Part model, mm, in its own coordinate system. A direction names the side the tool comes from. Coordinates: 2 decimals unless noted, no trailing zeros. Loops run counter-clockwise (first coordinate to the right, second up) from the corner with the lowest first, then second, coordinate; pieces in that order, holes last. Notation, with made-up numbers: (83, 11.5) - (127, 11.5) arc R14 ccw to (127, 17.5) - close; hole circle Ø6 at (53.5, -19.5). An arc over 180 degrees is marked (long way). Answer as CSV lines item,"result".
from build123d import *

# Parameters (mm, degrees)
SKETCH1_R           = 1.625
BOSS_EXTRUDE1_DEPTH = 5.842


with BuildPart() as part:
    # Sketch1 → Boss-Extrude1 (new body)
    with BuildSketch(Plane(origin=(0, 0, 0), x_dir=(1, 0, 0), z_dir=(0, 1, 0))):
        with BuildLine():
            Line((-23.368, 3.4), (-9.921693404, 3.4))
            ThreePointArc((-9.921693404, 3.4), (-7.818582155, 3.863820652), (-6.105657479, 5.169230769))
            ThreePointArc((-6.105657479, 5.169230769), (8, 0), (-6.105657479, -5.169230769))
            ThreePointArc((-6.105657479, -5.169230769), (-7.818582155, -3.863820652), (-9.921693404, -3.4))
            Line((-9.921693404, -3.4), (-23.368, -3.4))
            ThreePointArc((-23.368, -3.4), (-26.768, 0), (-23.368, 3.4))
        make_face()
        with Locations((-19.304, 0)):
            Circle(SKETCH1_R, mode=Mode.SUBTRACT)
        with Locations((-23.368, 0)):
            Circle(SKETCH1_R, mode=Mode.SUBTRACT)
    extrude(amount=BOSS_EXTRUDE1_DEPTH)


solid = part.part
Q1. Wall check: L1, parallel to X at y = 2.95, z = 0; L2, parallel to Z at x = -10, y = 5.55; L3, parallel to Z at x = -24, y = 0.45. Give the ranges that are in metal, low to high.
Results:
L1,"x = -26.77 to -24.99, -21.74 to -20.93, -17.68 to 8"
L2,"z = -3.4 to 3.4"
L3,"z = -3.34 to -1.5, 1.5 to 3.34"
Q2. Which spindle directions (+Z, -Z, +X, -X, +Y, -Y) get a long thin tool onto all of the face, cutting with end or side? Do faces 1 (the face through (-17, 3, 3.4)), 2 (the face through (-5, 5.842, 0)). Say none if no direction does.
Results:
face 1,"+Z, -X, +Y, -Y"
face 2,"+Z, -Z, +X, -X, +Y"
Q3. Two-plate mould, pull along X, no slides. Class faces 3 (the face through (-17, 3, -3.4)), 4 (the face through (-26.767, 2.88, 0.075)), 5 (the face through (-20.927, 2.88, -0.071)), 6 (the face through (8, 3, 0)): released by +X, released by -X, zero draft, split by the parting line, or undercut.
Results:
face 3,"zero draft"
face 4,"released by -X"
face 5,"undercut"
face 6,"split by the parting line"
Q4. Flat gauge pins, fed straight in: pin 1 (2 mm diameter, centred on x = -1.5, y = 3, fed in from +Z); pin 2 (1.5 mm diameter, centred on x = -12.5, y = 4, fed in from +Z); pin 3 (1.5 mm diameter, centred on y = 1.5, z = 3, fed in from +X). Where does each tip first touch, or does it go through?
Results:
pin 1,"stops at z = 7.98"
pin 2,"stops at z = 3.4"
pin 3,"stops at x = 7.68"
Q5. Saw through at C-C (x = -11.5). Give the cut face in (y, z).
Results:
outline,"(0, -3.4) - (5.84, -3.4) - (5.84, 3.4) - (0, 3.4) - close"
Q6. Saw through at B-B (y = 5.05). Give the cut face in (x, z) (3 decimals).
Results:
outline,"(-23.368, -3.4) - (-9.922, -3.4) arc R5 cw to (-6.106, -5.169) arc R8 ccw (long way) to (-6.106, 5.169) arc R5 cw to (-9.922, 3.4) - (-23.368, 3.4) arc R3.4 ccw to start; hole circle Ø3.25 at (-23.368, 0); hole circle Ø3.25 at (-19.304, 0)"
Q7. Saw through at D-D (z = 6.5). Give the cut face in (x, y), then the cut area to 3 significant figures.
Results:
outline,"(-4.66, 0) - (4.66, 0) - (4.66, 5.84) - (-4.66, 5.84) - close"
area,"54.5 mm^2"
Q8. Saw through at A-A (z = 0). Give the cut face in (x, y).
Results:
outline,"(-26.77, 0) - (-24.99, 0) - (-24.99, 5.84) - (-26.77, 5.84) - close; (-21.74, 0) - (-20.93, 0) - (-20.93, 5.84) - (-21.74, 5.84) - close; (-17.68, 0) - (8, 0) - (8, 5.84) - (-17.68, 5.84) - close"
